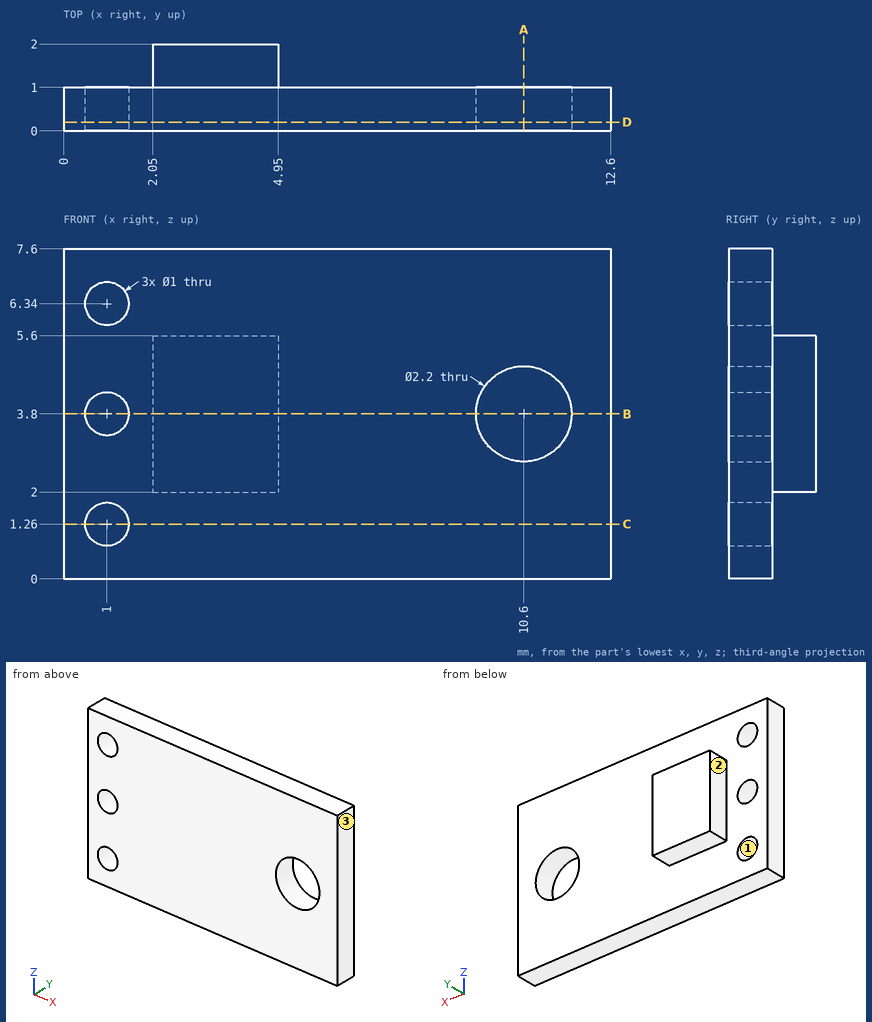
The drawing under review shows one solid part. Ordinate dimensions are in mm from its lowest x, y, z. Coordinates: 2 decimals unless noted, no trailing zeros. Order: outer loops, then holes, each group sorted by start corner. A loop starts at its lowest first (then second) coordinate and runs counter-clockwise, first axis right, second up. Notation, with made-up numbers: (52, 17.5) -> (58, 17.5) arc R23 ccw to (58, 26.5) -> close; hole circle Ø6 at (-4.75, 5.5). An arc over 180 degrees is marked (long way). Answer in a Markdown table with one row per item. Add a question column.
Item 1: We need section D-D on y = 0.2. Write out the cut boundary in (x, z).
Item 2: We need section A-A on x = 10.6. Write out the cut boundary in (y, z).
Item 3: Clearance check with flat-ended pins moving along their axes: pin 1 (2 mm diameter, centred on x = 10.6, z = 3.8, fed in from -Y); pin 2 (1.5 mm diameter, centred on x = 10.5, z = 4.5, fed in from +Y). State where each tip first meets the part, or that it passes through.
Item 4: We need section B-B on z = 3.8. Write out the cut boundary in (x, y), plus the area to 3 significant figures.
Item 5: To check wall thickness, follow probe 1 along X at (y, z) = (0.7, 3.8); probe 2 along Z at (x, y) = (1, 0.5); probe 3 along Z at (x, y) = (10.6, 0.6). State the ranges of each line that lie inside material, in increasing order.
Item 6: We need section C-C on z = 1.26. Write out the cut boundary in (x, y).
Item 7: Mouldability with a two-part tool opening along X and no side actions: class the marked faces 1, 2 and 3 as +X half, -X half, draft (parallel to the pull), parting line (faces both ways), or undercut.
Final values:
| question | item | result |
|---|---|---|
| 1 | outline | (0, 0) -> (12.6, 0) -> (12.6, 7.6) -> (0, 7.6) -> close; hole circle Ø1 at (1, 1.26); hole circle Ø1 at (1, 3.8); hole circle Ø1 at (1, 6.34); hole circle Ø2.2 at (10.6, 3.8) |
| 2 | outline | (0, 0) -> (1, 0) -> (1, 2.7) -> (0, 2.7) -> close; (0, 4.9) -> (1, 4.9) -> (1, 7.6) -> (0, 7.6) -> close |
| 3 | pin 1 | passes through |
| 3 | pin 2 | stops at y = 1 |
| 4 | outline | (0, 0) -> (0.5, 0) -> (0.5, 1) -> (0, 1) -> close; (1.5, 0) -> (9.5, 0) -> (9.5, 1) -> (4.95, 1) -> (4.95, 2) -> (2.05, 2) -> (2.05, 1) -> (1.5, 1) -> close; (11.7, 0) -> (12.6, 0) -> (12.6, 1) -> (11.7, 1) -> close |
| 4 | area | 12.3 mm2 |
| 5 | probe 1 | x = 0 to 0.5, 1.5 to 9.5, 11.7 to 12.6 |
| 5 | probe 2 | z = 0 to 0.76, 1.76 to 3.3, 4.3 to 5.84, 6.84 to 7.6 |
| 5 | probe 3 | z = 0 to 2.7, 4.9 to 7.6 |
| 6 | outline | (0, 0) -> (0.5, 0) -> (0.5, 1) -> (0, 1) -> close; (1.5, 0) -> (12.6, 0) -> (12.6, 1) -> (1.5, 1) -> close |
| 7 | face 1 | undercut |
| 7 | face 2 | -X half |
| 7 | face 3 | +X half |
